Verification items for this drawing (mm, ordinates from the low corner). A direction names the side the tool comes from. Round coordinates to 2 decimals unless told otherwise and drop trailing zeros. Order: outer loops, then holes, each group sorted by start corner. A loop starts at its lowest first (then second) coordinate and runs counter-clockwise, first axis right, second up. Notation, with made-up numbers: M 0,-10.5 L 50,-10.5 A27 cw 50,12.5 Z; hole C 84,-39.75 d1. An arc over 180 degrees is marked long. One line per item, written item: value. Start each with the question number.
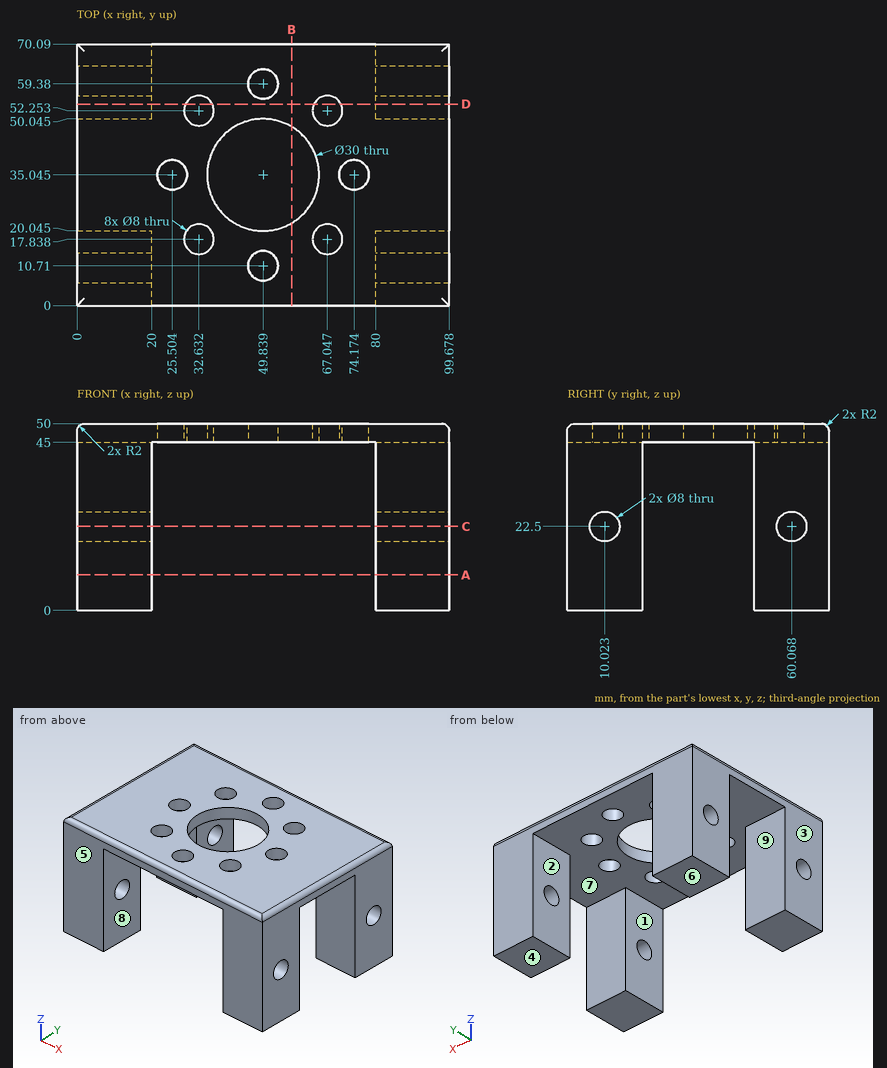
1. Section check C-C (z = 22.5). Give the number of separate pieces and of enclosed holes in the cut face.
2. Depth check by flat-ended pin: pin 1 (1 mm diameter, centred on x = 56.5, y = 55, fed in from -Z); pin 2 (6.5 mm diameter, centred on y = 60.07, z = 22.5, fed in from -X). Enter the tip coordinate at first touch or a pass-through.
3. Draft check along X on the marked faces 1, 2, 3 and 4. Enter one of: released by +X, released by -X, zero draft, split by the parting line, or undercut.
4. Section check A-A (z = 9.5). Record the cut outline in (x, y) (1 decimal).
5. Section check B-B (x = 57.5). Record the cut outline in (y, z).
6. Scan lines: line 1 along Y through (x, z) = (67.5, 47.5); line 2 along X through (y, z) = (66.5, 5.5); line 3 along Y through (x, z) = (92.5, 22.5) (1 decimal). Record each from-to range of solid material in increasing order.
7. Tool access check on the marked faces 5, 6, 7, 8 and 9. Record the directions out of +Z, -Z, +X, -X, +Y, -Y that give a thin tool (end or side, any length) a straight path to the whole face; none if there is none.
8. Section check D-D (y = 54). Record the cut outline in (x, z) (1 decimal).
Geometry check:
1. separate pieces: 8
1. enclosed holes: 0
2. pin 1: stops at z = 45
2. pin 2: passes through
3. face 1: undercut
3. face 2: undercut
3. face 3: released by -X
3. face 4: zero draft
4. outline: M 0,0 L 20,0 L 20,20 L 0,20 Z; M 0,50 L 20,50 L 20,70.1 L 0,70.1 Z; M 80,0 L 99.7,0 L 99.7,20 L 80,20 Z; M 80,50 L 99.7,50 L 99.7,70.1 L 80,70.1 Z
5. outline: M 0,45 L 22.15,45 L 22.15,50 L 2,50 A2 ccw 0,48 Z; M 47.94,45 L 70.09,45 L 70.09,48 A2 ccw 68.09,50 L 47.94,50 Z
6. line 1: y = 0 to 13.86, 21.81 to 48.28, 56.23 to 70.09
6. line 2: x = 0 to 20, 80 to 99.68
6. line 3: y = 0 to 6, 14 to 20, 50 to 56.1, 64.1 to 70.1
7. face 5: +Z, -Z, +X, -X, -Y
7. face 6: -Z, +X, -X, +Y, -Y
7. face 7: -Z
7. face 8: -Z, +Y, -Y
7. face 9: -Z, +X, -X
8. outline: M 0,0 L 20,0 L 20,45 L 29,45 L 29,50 L 2,50 A2 ccw 0,48 Z; M 36.2,45 L 63.4,45 L 63.4,50 L 36.2,50 Z; M 70.6,45 L 80,45 L 80,0 L 99.7,0 L 99.7,48 A2 ccw 97.7,50 L 70.6,50 Z
